The listing builds one solid part. Answer for the finished solid, in the listing's coordinates (mm). Face numbers are marked on the shaded views. A direction names the side the tool comes from. Coordinates: 2 decimals unless noted, no trailing zeros. Loops run counter-clockwise (first coordinate to the right, second up) from the corner with the lowest first, then second, coordinate; pieces in that order, holes last. Notation, with made-up numbers: (-17.5, -20.75) -> (-10.5, -20.75) arc R23 cw to (-10.5, 10.25) -> close; hole circle Ø11 at (62, 44.25). An arc over 180 degrees is marked (long way). Answer in a Markdown table with one row per item.
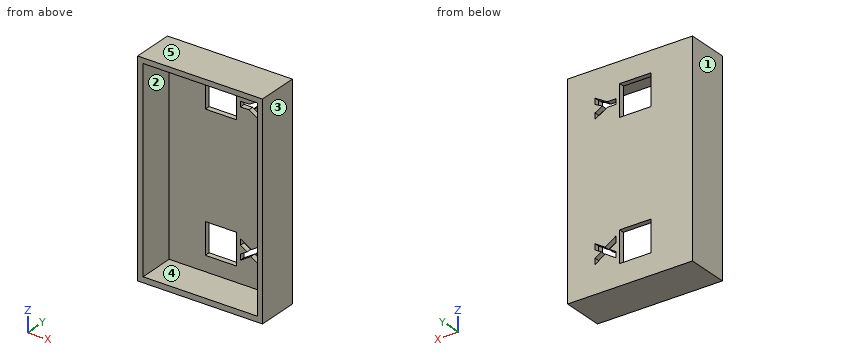
Autodesk Inventor part; units mm, degrees
ref_plane "YZ Plane" through (0, 0, 0) normal (1, 0, 0) x (0, 1, 0)
ref_plane "XZ Plane" through (0, 0, 0) normal (0, 1, 0) x (-1, 0, 0)
ref_plane "XY Plane" through (0, 0, 0) normal (0, 0, 1) x (1, 0, 0)
sketch "Sketch1" plane through (0, 0, 0) normal (0, 1, 0) x (-1, 0, 0)
  line L0 (0, 0) -> (76.2, 0)
  line L1 (76.2, 0) -> (76.2, -127)
  line L2 (76.2, -127) -> (0, -127)
  line L3 (0, -127) -> (0, 0)
  dimension "d0" = 76.2
  dimension "d1" = 127
extrude "Extrusion1" add sketch "Sketch1" along normal blind 25.4
sketch "Sketch2" plane through (0, 0, 0) normal (0, -1, 0) x (1, 0, 0)
  line L0 (-3.1691, -3.1691) -> (-72.8902, -3.1691)
  line L1 (-72.8902, -3.1691) -> (-72.8902, -123.5964)
  line L2 (-72.8902, -123.5964) -> (-3.1691, -123.5964)
  line L3 (-3.1691, -123.5964) -> (-3.1691, -3.1691)
  point P0 (0, 0)
extrude "Extrusion2" cut sketch "Sketch2" against normal blind 22.225
sketch "Sketch3" plane through (0, 25.4, 0) normal (0, 1, 0) x (1, 0, 0)
  line L0 (-50.8, 12.7) -> (-31.75, 12.7)
  line L1 (-31.75, 12.7) -> (-31.75, 31.75)
  line L2 (-31.75, 31.75) -> (-50.8, 31.75)
  line L3 (-50.8, 31.75) -> (-50.8, 12.7)
  line L4 (-50.8, 95.25) -> (-31.75, 95.25)
  line L5 (-31.75, 95.25) -> (-31.75, 114.3)
  line L6 (-31.75, 114.3) -> (-50.8, 114.3)
  line L7 (-50.8, 114.3) -> (-50.8, 95.25)
  line L8 (-76.2, 127) -> (-76.2, 0)
  line L9 (-76.2, 0) -> (0, 0)
  line L10 (0, 127) -> (-76.2, 127)
  dimension "d6" = 19.05
  dimension "d7" = 19.05
  dimension "d8" = 25.4
  dimension "d9" = 25.4
  dimension "d10" = 19.05
  dimension "d11" = 19.05
  dimension "d12" = 12.7
  dimension "d13" = 12.7
extrude "Extrusion3" cut sketch "Sketch3" against normal blind 22.225
sketch "Sketch4" plane through (0, 25.4, 0) normal (0, 1, 0) x (1, 0, 0)
  line L0 (-13.7708, 110.3112) -> (-13.7708, 97.845) construction
  line L1 (-13.7708, 97.845) -> (-32.3251, 97.845) construction
  line L2 (-32.3251, 97.845) -> (-32.3251, 110.3112) construction
  line L3 (-32.3251, 110.3112) -> (-13.7708, 110.3112) construction
  line L4 (-12.0313, 30.7306) -> (-12.0313, 13.191) construction
  line L5 (-12.0313, 13.191) -> (-34.0646, 13.191) construction
  line L6 (-34.0646, 13.191) -> (-34.0646, 30.7306) construction
  line L7 (-34.0646, 30.7306) -> (-12.0313, 30.7306) construction
  line L8 (-29.3979, 98.0986) -> (-29.3979, 101.783)
  line L9 (-29.3979, 101.783) -> (-25.3533, 104.2325)
  line L10 (-25.3533, 104.2325) -> (-29.3979, 106.7333)
  line L11 (-29.3979, 106.7333) -> (-29.3979, 110.2634)
  line L12 (-29.3979, 110.2634) -> (-23.0068, 106.1364)
  line L13 (-23.0068, 106.1364) -> (-16.6979, 110.0987)
  line L14 (-16.6979, 110.0987) -> (-16.6979, 106.4143)
  line L15 (-16.6979, 106.4143) -> (-20.5367, 104.1192)
  line L16 (-20.5367, 104.1192) -> (-16.6979, 101.7624)
  line L17 (-16.6979, 101.7624) -> (-16.6979, 98.2324)
  line L18 (-16.6979, 98.2324) -> (-22.873, 102.2153)
  line L19 (-22.873, 102.2153) -> (-29.3979, 98.0986)
  line L20 (-16.6979, 16.0996) -> (-24.0977, 20.4839)
  line L21 (-24.0977, 20.4839) -> (-29.3979, 20.4839)
  line L22 (-29.3979, 20.4839) -> (-29.3979, 23.6743)
  line L23 (-29.3979, 23.6743) -> (-24.2521, 23.6743)
  line L24 (-24.2521, 23.6743) -> (-16.6979, 28.1307)
  line L25 (-16.6979, 28.1307) -> (-16.6979, 24.4977)
  line L26 (-16.6979, 24.4977) -> (-21.2263, 22.0174)
  line L27 (-21.2263, 22.0174) -> (-16.6979, 19.6194)
  line L28 (-16.6979, 19.6194) -> (-16.6979, 16.0996)
  point P0 (0, 0)
extrude "Extrusion4" cut sketch "Sketch4" against normal blind 25.4
properties part number "gamebox"
Item 1: A cutting plane is placed at B-B, the plane y = 2. Determine the outline of the cut face in (x, z), plus the area to 3 significant figures.
Findings below:
| item | result |
|---|---|
| outline | (-76.2, -127) -> (0, -127) -> (0, 0) -> (-76.2, 0) -> close; hole (-72.89, -123.6) -> (-3.17, -123.6) -> (-3.17, -3.17) -> (-72.89, -3.17) -> close |
| area | 1,280 mm2 |
Item 2: A cutting plane is placed at C-C, the plane z = -88. Determine the outline of the cut face in (x, y) (3 decimals).
Findings below:
| item | result |
|---|---|
| outline | (-76.2, 0) -> (-72.89, 0) -> (-72.89, 22.225) -> (-3.169, 22.225) -> (-3.169, 0) -> (0, 0) -> (0, 25.4) -> (-76.2, 25.4) -> close |
Item 3: A tool of negligible diameter and unlimited length cuts with its end or side. For the marked faces 1 and 2, from which of +Z, -Z, +X, -X, +Y, -Y can it reach the whole face along a straight path? Write none if from no direction.
Findings below:
| item | result |
|---|---|
| face 1 | +Z, -Z, -X, +Y, -Y |
| face 2 | -Y |
Item 4: A cutting plane is placed at A-A, the plane x = -49.5. Determine the outline of the cut face in (y, z) (3 decimals), plus the area to 3 significant figures.
Findings below:
| item | result |
|---|---|
| outline | (0, -127) -> (25.4, -127) -> (25.4, -114.3) -> (22.225, -114.3) -> (22.225, -123.596) -> (0, -123.596) -> close; (0, -3.169) -> (22.225, -3.169) -> (22.225, -12.7) -> (25.4, -12.7) -> (25.4, 0) -> (0, 0) -> close; (22.225, -95.25) -> (25.4, -95.25) -> (25.4, -31.75) -> (22.225, -31.75) -> close |
| area | 428 mm2 |
Item 5: A cutting plane is placed at D-D, the plane x = -67. Determine the outline of the cut face in (y, z) (3 decimals), plus the area to 3 significant figures.
Findings below:
| item | result |
|---|---|
| outline | (0, -127) -> (25.4, -127) -> (25.4, 0) -> (0, 0) -> (0, -3.169) -> (22.225, -3.169) -> (22.225, -123.596) -> (0, -123.596) -> close |
| area | 549 mm2 |
Item 6: Find the intervals of material crossed by probe 1 along Z at (x, y) = (-46.5, 23.75); probe 2 along X at (y, z) = (13, -37); probe 3 along Z at (x, y) = (-61, 2.5), in increasing order.
Findings below:
| item | result |
|---|---|
| probe 1 | z = -127 to -114.3, -95.25 to -31.75, -12.7 to 0 |
| probe 2 | x = -76.2 to -72.89, -3.17 to 0 |
| probe 3 | z = -127 to -123.6, -3.17 to 0 |
Item 7: Determine the mould class of the marked faces 3, 4 and 5 for opening direction X: +X half, -X half, draft (parallel to the pull), parting line (faces both ways), or undercut.
Findings below:
| item | result |
|---|---|
| face 3 | +X half |
| face 4 | undercut |
| face 5 | draft |
Item 8: Flat-ended cylindrical pins translate along their axes: pin 1 Ø4 at (x, z) = (-43, -46.5) entering from -Y (3 decimals); pin 2 Ø1 at (y, z) = (23, -100.5) entering from +X. Find the tip coordinate at first contact, or state that the pin passes through.
Findings below:
| item | result |
|---|---|
| pin 1 | stops at y = 22.225 |
| pin 2 | stops at x = 0 |
